Here's how the part is built. I have some questions about the finished solid (model axes, mm). A direction names the side the tool comes from. Coordinates: 2 decimals unless noted, no trailing zeros. Write each loop counter-clockwise with the first axis right and the second up, starting at its lowest first coordinate (ties: lowest second). Pieces come first, ordered by that corner, then holes. Notation, with made-up numbers: (22.25, 33.25) -> (48.25, 33.25) arc R20 ccw to (48.25, 46.25) -> close; hole circle Ø6 at (48, 68). An arc over 180 degrees is marked (long way). Use a Markdown table: item, result. Add a question column.
Item 1: Imagine slicing it at A-A, the plane y = 0. Write out the boundary of the cut face in (x, z), and give its area (3 significant figures).
Item 2: Imagine slicing it at B-B, the plane z = 17.75. Write out the boundary of the cut face in (x, y), and give its area (3 significant figures).
Item 3: On a 3-axis mill with a long thin cutter (end or side, diameter ignored), from which of +Z, -Z, +X, -X, +Y, -Y can I reach the whole of each face in a straight line? I mean faces 1 (the flat face through (2.54, 4, 10)), 2 (the flat face through (4, -4, 20.32)), 3 (the cylindrical face through (-1.606, 7.233, 10.281)). Say none if no direction works.
Item 4: Will these pins go through, and if not, where does the flat tip stop? pin 1 Ø1.9 at (y, z) = (4, 6) entering from -X; pin 2 Ø4 at (y, z) = (4.5, 6) entering from +X; pin 3 Ø4 at (x, z) = (-1.5, 9.5) entering from -Y.
Item 5: If I drill on line 1 along Z through (x, y) = (8, 3.5); line 2 along X through (y, z) = (4.25, 10); line 3 along Y through (x, z) = (-1.75, 2), over which ranges is the centre line in solid material (lowest first)? Write a range as from..to.
Item 6: If we mould it in two halves opening along Z, with no side actions, what happens to faces 4 (the flat face through (3, -7, 18.546)), 5 (the flat face through (4, -4, 0)), 6 (the flat face through (6.35, 0, 10))? For each: pulls with the +Z half, pulls with the -Z half, needs draft (parallel to the pull), parting line crosses it, or undercut.
```python
from build123d import *

# Parameters (mm, degrees)
F0_R     = 8.89
F1_DEPTH = 20.32
F3_DEPTH = 20.32
F4_W     = 3.678773
F4_H     = 16.764444


with BuildPart() as f1:
    # F0 (on Top) → F1 (new body)
    with BuildSketch(Plane.XY):
        Circle(F0_R)
    extrude(amount=F1_DEPTH)

    # F2 (on face) → F3 (cut)
    with BuildSketch(Plane.XY.offset(20.32)):
        Polygon((-2.526941, -6.35), (0, -6.35), (2.54, -6.35), (2.54, -2.54), (6.35, -2.54), (6.35, 0), (6.35, 2.540121), (2.54, 2.540121), (2.54, 6.345605), (0, 6.345605), (-2.54, 6.345605), (-2.54, 2.540121), (-6.35, 2.540121), (-6.35, 0), (-6.35, -2.54), (-2.54, -2.54), align=None)
    extrude(amount=-F3_DEPTH, mode=Mode.SUBTRACT)

    # F4 (on Front) → F5 (revolve, cut)
    with BuildSketch(Plane.XZ):
        with Locations((9.249083, 10.164065)):
            Rectangle(F4_W, F4_H)
    revolve(axis=Axis((0, 0, 10.164065), (0, 0, -1)), mode=Mode.SUBTRACT)


solid = f1.part
```
Ans:
| question | item | result |
|---|---|---|
| 1 | outline | (-8.89, 0) -> (-6.35, 0) -> (-6.35, 20.32) -> (-8.89, 20.32) -> (-8.89, 18.55) -> (-7.41, 18.55) -> (-7.41, 1.78) -> (-8.89, 1.78) -> close; (6.35, 0) -> (8.89, 0) -> (8.89, 1.78) -> (7.41, 1.78) -> (7.41, 18.55) -> (8.89, 18.55) -> (8.89, 20.32) -> (6.35, 20.32) -> close |
| 1 | area | 53.6 mm^2 |
| 2 | outline | circle Ø14.82 at (0, 0); hole (-6.35, -2.54) -> (-2.54, -2.54) -> (-2.53, -6.35) -> (2.54, -6.35) -> (2.54, -2.54) -> (6.35, -2.54) -> (6.35, 2.54) -> (2.54, 2.54) -> (2.54, 6.35) -> (-2.54, 6.35) -> (-2.54, 2.54) -> (-6.35, 2.54) -> close |
| 2 | area | 69.3 mm^2 |
| 3 | face 1 | +Z, -Z |
| 3 | face 2 | +Z, +X, -X, +Y, -Y |
| 3 | face 3 | none |
| 4 | pin 1 | stops at x = -6.75 |
| 4 | pin 2 | stops at x = 6.98 |
| 4 | pin 3 | stops at y = -7.41 |
| 5 | line 1 | z = 0..1.78, 18.55..20.32 |
| 5 | line 2 | x = -6.07..-2.54, 2.54..6.07 |
| 5 | line 3 | y = -7.2..-6.35, 6.35..7.2 |
| 6 | face 4 | undercut |
| 6 | face 5 | pulls with the -Z half |
| 6 | face 6 | needs draft |
